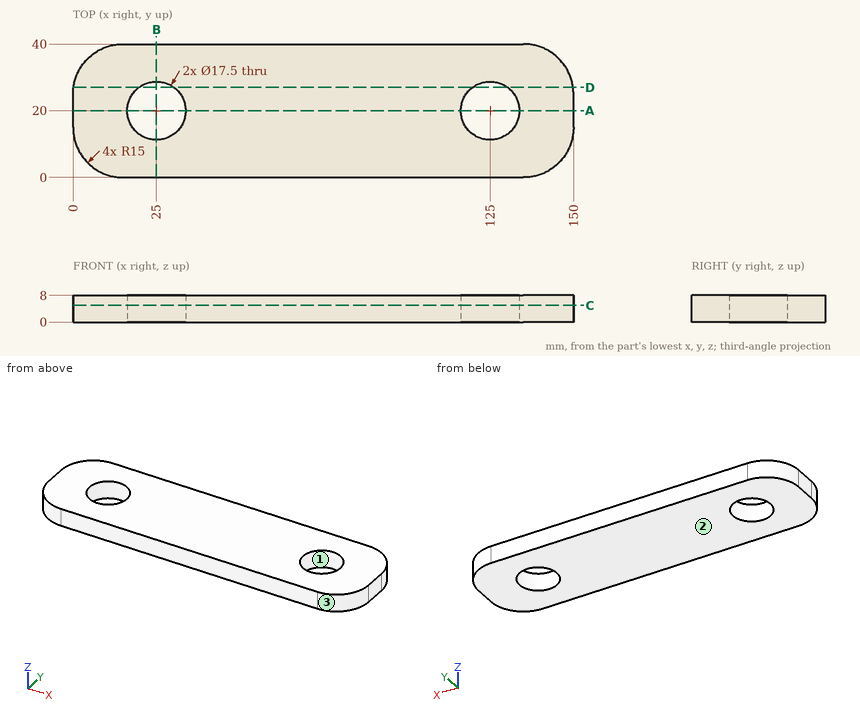
Check sheet for the drawn part. Datum: minimum x, y, z corner. Units: mm. Coordinates: 2 decimals unless noted, no trailing zeros. Loops run counter-clockwise (first coordinate to the right, second up) from the corner with the lowest first, then second, coordinate; pieces in that order, holes last. Notation, with made-up numbers: (-26, -10.75) - (33, -10.75) arc R25 ccw to (33, 17.25) - close; hole circle Ø3 at (8.5, 59.5). An arc over 180 degrees is marked (long way). Put each result on its own line as item: value.
Item 1: Draft check along Y on the marked faces 1, 2 and 3. Enter one of: pulls with the +Y half, pulls with the -Y half, needs draft (parallel to the pull), parting line crosses it, or undercut.
Conclusion:
face 1: undercut
face 2: needs draft
face 3: pulls with the -Y half
Item 2: Section check A-A (y = 20). Enter the section's corners in (x, z).
Conclusion:
outline: (0, 0) - (16.25, 0) - (16.25, 8) - (0, 8) - close; (33.75, 0) - (116.25, 0) - (116.25, 8) - (33.75, 8) - close; (133.75, 0) - (150, 0) - (150, 8) - (133.75, 8) - close
Item 3: Gauge pin test, flat ends, axial feed: pin 1 Ø1 at (y, z) = (6, 6.5) entering from -X; pin 2 Ø1.5 at (y, z) = (5.5, 4) entering from -X; pin 3 Ø3 at (y, z) = (29.5, 2.5) entering from +X. Record the tip position at first contact, or that the pin passes through.
Conclusion:
pin 1: stops at x = 2.64
pin 2: stops at x = 2.82
pin 3: stops at x = 149.7
Item 4: Section check C-C (z = 5). Enter the section's corners in (x, y).
Conclusion:
outline: (0, 15) arc R15 ccw to (15, 0) - (135, 0) arc R15 ccw to (150, 15) - (150, 25) arc R15 ccw to (135, 40) - (15, 40) arc R15 ccw to (0, 25) - close; hole circle Ø17.5 at (25, 20); hole circle Ø17.5 at (125, 20)
Item 5: Scan lines: line 1 along Y through (x, z) = (25, 5.5); line 2 along X through (y, z) = (16.5, 2.25); line 3 along X through (y, z) = (15, 3.5). Record each from-to range of solid material in increasing order.
Conclusion:
line 1: y = 0 to 11.25, 28.75 to 40
line 2: x = 0 to 16.98, 33.02 to 116.98, 133.02 to 150
line 3: x = 0 to 17.82, 32.18 to 117.82, 132.18 to 150
Item 6: Section check B-B (x = 25). Enter the section's corners in (y, z).
Conclusion:
outline: (0, 0) - (11.25, 0) - (11.25, 8) - (0, 8) - close; (28.75, 0) - (40, 0) - (40, 8) - (28.75, 8) - close
Item 7: Section check D-D (y = 27). Enter the section's corners in (x, z), then the cut area to 3 significant figures.
Conclusion:
outline: (0.13, 0) - (19.75, 0) - (19.75, 8) - (0.13, 8) - close; (30.25, 0) - (119.75, 0) - (119.75, 8) - (30.25, 8) - close; (130.25, 0) - (149.87, 0) - (149.87, 8) - (130.25, 8) - close
area: 1,030 mm2
